Autodesk Fusion 360 part; units mm, degrees
sketch "Sketch1" plane through (0, 0, 0) normal (0, 0, 1) x (1, 0, 0)
  line L0 (-3, -13) -> (-8, -13)
  line L1 (-8, -13) -> (-8, 5)
  line L2 (-8, 5) -> (8, 5)
  line L3 (8, 5) -> (8, -13)
  line L4 (8, -13) -> (3, -13)
  line L5 (3, -13) -> (3, 0)
  line L6 (3, 0) -> (-3, 0)
  line L7 (-3, 0) -> (-3, -13)
  dimension "d1" = 6
  dimension "d2" = 5
  dimension "d3" = 5
  dimension "d4" = 5
  dimension "d6" = 13
extrude "Extrude1" add sketch "Sketch1" along normal blind 10 makes body 1
sketch "Sketch2" plane through (3, 0, 0) normal (-1, 0, 0) x (0, 0, 1)
  line L0 (0, 0) -> (0, -13)
  line L1 (0, -13) -> (10, -13)
  line L2 (10, -13) -> (10, 0)
  line L3 (10, 0) -> (0, 0)
  line L4 (8.45, -8.4919) -> (8.45, -4.5081)
  line L5 (8.45, -4.5081) -> (5, -2.5163)
  line L6 (5, -2.5163) -> (1.55, -4.5081)
  line L7 (1.55, -4.5081) -> (1.55, -8.4919)
  line L8 (1.55, -8.4919) -> (5, -10.4837)
  line L9 (5, -10.4837) -> (8.45, -8.4919)
  point P0 (5, -6.5)
  point P1 (5, 0)
  dimension "d9" = 3.45
  dimension "d10" = 6.5
extrude "Extrude2" cut sketch "Sketch2" against normal blind 3.2 contours L4 L5 L6 L7 L8 L9 bodies 1
hole "Hole1" at (3, -6.5, 5) direction (1, 0, 0) diameter 4.3 end through all bodies 1 1
sketch "Sketch3" plane through (0, 0, 0) normal (1, 0, 0) x (0, 0, -1)
  circle A0 centre (0, 0) radius 8
  line L0 (0, -3.9837) -> (3.45, -1.9919)
  line L1 (3.45, -1.9919) -> (3.45, 1.9919)
  line L2 (3.45, 1.9919) -> (0, 3.9837)
  line L3 (0, 3.9837) -> (-3.45, 1.9919)
  line L4 (-3.45, 1.9919) -> (-3.45, -1.9919)
  line L5 (-3.45, -1.9919) -> (0, -3.9837)
  circle A1 centre (0, 9) radius 1.75
  circle A2 centre (-4.1825, 7.9691) radius 1.75
  circle A3 centre (-7.4069, 5.1126) radius 1.75
  circle A4 centre (-8.9344, 1.0848) radius 1.75
  circle A5 centre (-8.4151, -3.1914) radius 1.75
  circle A6 centre (-5.9681, -6.7366) radius 1.75
  circle A7 centre (-2.1538, -8.7385) radius 1.75
  circle A8 centre (2.1538, -8.7385) radius 1.75
  circle A9 centre (5.9681, -6.7366) radius 1.75
  circle A10 centre (8.4151, -3.1914) radius 1.75
  circle A11 centre (8.9344, 1.0848) radius 1.75
  circle A12 centre (7.4069, 5.1126) radius 1.75
  circle A13 centre (4.1825, 7.9691) radius 1.75
  dimension "d16" = 16
  dimension "d17" = 3.45
  dimension "d18" = 3.5
  dimension "d19" = 9
  dimension "d21" = 360
extrude "Extrude3" add sketch "Sketch3" along normal blind 5 separate body contours A0 A1 A2 A3 A4 A5 A6 A7 A8 A9 A10 A11 A12 A13 | L0 L1 L2 L3 L4 L5 makes body 2
extrude "Extrude4" cut sketch "Sketch3" along normal blind 3 contours L0 L1 L2 L3 L4 L5 bodies 2
hole "Hole2" at (0, 0, 0) direction (-1, 0, 0) diameter 4.2 end through all bodies 2 2
sketch "Sketch4" plane through (0, 0, 10) normal (0, 0, 1) x (1, 0, 0)
  line L0 (-3, 0) -> (3, 0)
  line L1 (3, 0) -> (3, -13)
  line L2 (3, -13) -> (8, -13)
  line L3 (8, -13) -> (8, 5)
  line L4 (8, 5) -> (-8, 5)
  line L5 (-8, 5) -> (-8, -13)
  line L6 (-8, -13) -> (-3, -13)
  line L7 (-3, -13) -> (-3, 0)
  line L8 (-3, -12) -> (-4.2, -10.8)
  line L9 (-4.2, -10.8) -> (-3, -9.6)
  line L10 (-4.2, -8.1333) -> (-3, -6.9333)
  line L11 (-3, -9.3333) -> (-4.2, -8.1333)
  line L12 (-4.2, -5.4667) -> (-3, -4.2667)
  line L13 (-3, -6.6667) -> (-4.2, -5.4667)
  line L14 (-4.2, -2.8) -> (-3, -1.6)
  line L15 (-3, -4) -> (-4.2, -2.8)
  dimension "d29" = 1.2
  dimension "d30" = 1
  dimension "d33" = 0
  dimension "d34" = 8
extrude "Extrude5" cut sketch "Sketch4" along normal through all contours L7 L14 L15 | L7 L12 L13 | L7 L10 L11 | L7 L8 L9 bodies 1
fillet "Fillet2" radius 5 2 edges at (5.5, -13, 10) (5.5, -13, 0) on bodies 1
fillet "Fillet1" radius 4 3 edges at (-8, 5, 5) (8, 5, 5) (-8, -13, 5) on bodies 1
fillet "Fillet1" radius 1 2 edges at (-3, 0, 5) (3, 0, 5) on bodies 1
fillet "Fillet3" radius 1 26 edges at (0, 4.1185, 5.9666) (0, 2.8368, 7.4801) (0, 0.8739, 7.1971) (0, -0.9643, 7.9417) (0, -2.5709, 6.7789) (0, -4.5445, 6.5839) (0, -5.4267, 4.8076) (0, -7.0836, 3.7178) (0, -7.0393, 1.735) (0, -8, 0) (0, -7.0393, -1.735) (0, -7.0836, -3.7178) (0, -5.4267, -4.8076) (0, -4.5445, -6.5839) (0, -2.5709, -6.7789) (0, -0.9643, -7.9417) (0, 0.8739, -7.1971) (0, 2.8368, -7.4801) (0, 4.1185, -5.9666) (0, 5.9881, -5.305) (0, 6.4196, -3.3692) (0, 7.7675, -1.9145) (0, 7.25, 0) (0, 7.7675, 1.9145) (0, 6.4196, 3.3692) (0, 5.9881, 5.305) on bodies 2
hidden bodies 2
equation "d9 = ( 6.9 / 2 ) * 1 mm"
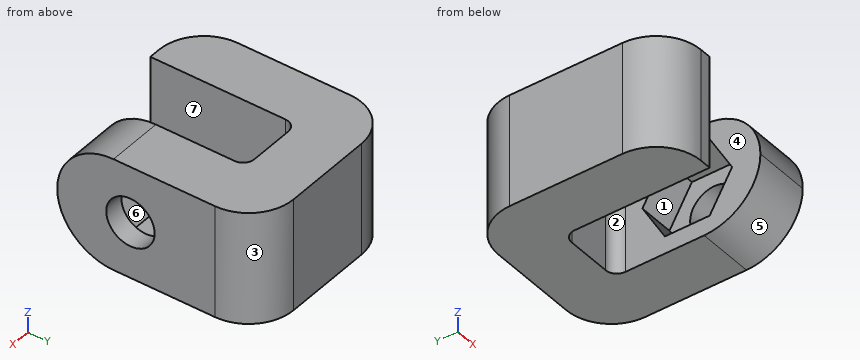
Design review of the part built by this model. Coordinates are the model's own, in mm. Face numbers are marked on the shaded views. A direction names the side the tool comes from. Give positions to 0.01 mm unless a question says otherwise; leave off trailing zeros. Order: outer loops, then holes, each group sorted by start corner. A loop starts at its lowest first (then second) coordinate and runs counter-clockwise, first axis right, second up. Notation, with made-up numbers: (43.5, 57.25) - (54.5, 57.25) arc R35 ccw to (54.5, 90.25) - close; hole circle Ø6 at (-2.5, 34.5). An arc over 180 degrees is marked (long way). Use CSV: the item, a comma, the result in double quotes. Start each with the question number.
Q1. For P1, Ø4, axis at x = 3, z = 1.5, coming from the -Y side; P2, Ø4, axis at x = 4.5, z = 4, coming from the +Y side; P3, Ø1.2, axis at x = 0.5, z = 5.5, coming from the -Y side, all flat-tipped, find the tip position at first contact; note any pin that passes through.
Q2. Draft analysis for pull direction Y (two halves, no side actions). For the marked faces 1, 2, 3 and 4, state which applies: pulls with the +Y half, pulls with the -Y half, needs draft (parallel to the pull), parting line crosses it, or undercut.
Q3. Take a section at B-B (y = -2). State the section outline as (x, z) points, and give its area (3 significant figures).
Q4. Take a section at A-A (y = -6.5). State the section outline as (x, z) points.
Q5. Machinability: for the marked faces 5, 6 and 7, which of the approach directions +Z, -Z, +X, -X, +Y, -Y give a long, thin tool a straight path to every point of the face, cutting with its end or side? Answer none if there is none.
Q6. For line 1 (X direction, y = -3, z = 3.5); line 2 (Z direction, x = 6.6, y = -6.5); line 3 (Y direction, x = 6.65, z = 5), list the stretches that pass through material, from the lowest coordinate up.
Q7. Take a section at C-C (z = 4.5). State the section outline as (x, y) points.
Calculated:
1,P1,"stops at y = -12.77"
1,P2,"stops at y = 5"
1,P3,"stops at y = 0"
2,face 1,"undercut"
2,face 2,"pulls with the -Y half"
2,face 3,"pulls with the +Y half"
2,face 4,"needs draft"
3,outline,"(-8, 0) - (-3, 0) - (-3, 10) - (-8, 10) - close; (3, 0) - (8, 0) - (8, 10) - (3, 10) - close"
3,area,"100 mm²"
4,outline,"(-8, 0) - (-3, 0) - (-3, 10) - (-8, 10) - close; (3, 0) - (8, 0) - (8, 2.85) - (6.2, 2.85) - (6.2, 1.55) - (3, 1.55) - close; (3, 8.45) - (6.2, 8.45) - (6.2, 7.15) - (8, 7.15) - (8, 10) - (3, 10) - close"
5,face 5,"-Z, +X, -Y"
5,face 6,"none"
5,face 7,"+Z, -Z, -Y"
6,line 1,"x = -8 to -3, 3 to 8"
6,line 2,"z = 0 to 2.85, 7.15 to 10"
6,line 3,"y = -13 to -8.65, -4.35 to 4"
7,outline,"(-8, -9) arc R4 ccw to (-4, -13) - (-3, -13) - (-3, -1) arc R1 cw to (-2, 0) - (2, 0) arc R1 cw to (3, -1) - (3, -2.8) - (6.2, -2.8) - (6.2, -4.41) - (8, -4.41) - (8, 1) arc R4 ccw to (4, 5) - (-4, 5) arc R4 ccw to (-8, 1) - close; (3, -12.98) - (8, -12.98) - (8, -8.59) - (6.2, -8.59) - (6.2, -10.2) - (3, -10.2) - close"
